Source: CAD feature listing. Evaluate the final solid. Frame: model axes, mm. Give positions to 0.01 mm unless a question says otherwise; leave off trailing zeros. Loops run counter-clockwise (first coordinate to the right, second up) from the corner with the lowest first, then second, coordinate; pieces in that order, holes last.
from build123d import *

# Parameters (mm, degrees)
RESSALTO_EXTRUS_O1_DEPTH = 3
CORTE_EXTRUS_O1_DEPTH    = 151.026697624
ESBO_O5_R                = 1.15
ESBO_O5_R_2              = 1.149998009
ESBO_O5_R_3              = 1.149993787
CORTE_EXTRUS_O3_DEPTH    = 128.178545465


with BuildPart() as part:
    # Esboço1 → Ressalto-extrusão1 (new body)
    with BuildSketch(Plane(origin=(0, 0, 0), x_dir=(1, 0, 0), z_dir=(0, 1, 0))):
        Polygon((-75, 0), (75, 0), (0, 129.9), align=None)
    extrude(amount=RESSALTO_EXTRUS_O1_DEPTH)

    # Esboço3 → Corte-extrusão1 (cut, through all)
    with BuildSketch(Plane(origin=(0, 3, 0), x_dir=(1, 0, 0), z_dir=(0, 1, 0))):
        Polygon((52.12820532, 0), (63.556663987, 19.819857975), (75, 0), align=None)
        Polygon((-52.141215794, 0), (-63.556663987, 19.819857975), (-75, 0), align=None)
        Polygon((-11.421585635, 110.117813679), (11.421585635, 110.117813679), (0, 129.9), align=None)
    extrude(amount=-CORTE_EXTRUS_O1_DEPTH, mode=Mode.SUBTRACT)

    # Esboço5 → Corte-extrusão3 (cut, through all)
    with BuildSketch(Plane(origin=(0, 3, 0), x_dir=(1, 0, 0), z_dir=(0, 1, 0))):
        with Locations(Location((-49.687989721, 4.250373636, 0), (0, 0, 270))):
            Circle(ESBO_O5_R)
        with Locations(Location((-58.687989721, 19.838830904, 0), (0, 0, 270))):
            Circle(ESBO_O5_R)
        with Locations(Location((58.661761519, 19.83730914, 0), (0, 0, 270))):
            Circle(ESBO_O5_R)
        with Locations(Location((49.661761519, 4.248851872, 0), (0, 0, 270))):
            Circle(ESBO_O5_R)
        with Locations(Location((-8.943534892, 105.865797451, 0), (0, 0, 270))):
            Circle(ESBO_O5_R_2)
        with Locations(Location((9.05637457, 105.866807251, 0), (0, 0, 270))):
            Circle(ESBO_O5_R_3)
    extrude(amount=-CORTE_EXTRUS_O3_DEPTH, mode=Mode.SUBTRACT)


solid = part.part
1) Cut plane C-C (z = -98). Return loops of the section in (x, y), and give its area (3 significant figures).
Checks:
outline: (-18.42, 0) - (18.42, 0) - (18.42, 3) - (-18.42, 3) - close
area: 111 mm2
2) Cut plane B-B (x = 35.5). Return loops of the section in (y, z), and give its area (3 significant figures).
Checks:
outline: (0, -68.41) - (3, -68.41) - (3, 0) - (0, 0) - close
area: 205 mm2
3) Ray query, probe 1 along Z at (x, y) = (-9, 1.45); probe 2 along X at (y, z) = (0.6, -4.5); probe 3 along Z at (x, y) = (45, 2.3). Return the intervals inside material, ascending.
Checks:
probe 1: z = -110.12 to -107.01, -104.72 to 0
probe 2: x = -54.73 to -50.81, -48.57 to 48.54, 50.78 to 54.72
probe 3: z = -51.96 to 0
4) Contact query for flat-ended pins moving along their axis: P1, Ø2.5, axis at x = 58.66, z = -19.84, coming from the +Y side; P2, Ø2, axis at x = 49.66, z = -4.25, coming from the -Y side; P3, Ø1, axis at y = 0.5, z = -26, coming from the +X side; P4, Ø1, axis at x = 25, y = 0.5, coming from the -Z side. Output: stop coordinate, or through.
Checks:
P1: stops at y = 3
P2: passes through
P3: stops at x = 60.28
P4: stops at z = -87.47
5) Pull-direction query (Y, two-part tool) for faces 1 (the flat face through (0, 2, -110.118)), 2 (the flat face through (-1, 0, -44)), 3 (the flat face through (-1, 3, -44)); classes: released by +Y, released by -Y, zero draft, split by the parting line, or undercut.
Checks:
face 1: zero draft
face 2: released by -Y
face 3: released by +Y
6) Cut plane A-A (y = 1.3). Return loops of the section in (x, z), and give its area (3 significant figures).
Checks:
outline: (-63.56, -19.82) - (-11.42, -110.12) - (11.42, -110.12) - (63.56, -19.82) - (52.13, 0) - (-52.14, 0) - close; hole circle Ø2.3 at (-58.69, -19.84); hole circle Ø2.3 at (-49.69, -4.25); hole circle Ø2.3 at (-8.94, -105.87); hole circle Ø2.3 at (9.06, -105.87); hole circle Ø2.3 at (49.66, -4.25); hole circle Ø2.3 at (58.66, -19.84)
area: 9,040 mm2
